Geometry: final body of the model. Coordinates: model frame, mm. Face numbers are marked on the shaded views. A direction names the side the tool comes from. Coordinates: 2 decimals unless noted, no trailing zeros. Write each loop counter-clockwise with the first axis right and the second up, starting at its lowest first coordinate (ties: lowest second). Pieces come first, ordered by that corner, then holes. Notation, with made-up numbers: (53.25, 65.25) - (72.25, 65.25) arc R9 cw to (72.25, 75.25) - close; hole circle Ø10 at (88.25, 8). An arc over 180 degrees is marked (long way). Answer as a JSON object with one key per item and string values. Group by question number.
Item 1: Section B-B on y = -16.25. Return loops of the section in (x, z), and give its area (3 significant figures).
Item 2: Section C-C on x = 32.5. Return loops of the section in (y, z).
Item 3: Line query: line 1 along Z through (x, y) = (21, -9); line 2 along Y through (x, z) = (87.5, 25); line 3 along X through (y, z) = (-10.25, 27.75). Output: solid intervals per line, ascending. Write a range as from..to.
Item 4: Section A-A on z = 7.5. Return loops of the section in (x, y).
Item 5: Set-up query: the marked faces 1, 2 and 3. Return all of +Z, -Z, +X, -X, +Y, -Y with unobstructed straight access to the full face (end or side cutting, diameter ignored); none if empty.
Item 6: First-contact query: pin 1 Ø4 at (x, y) = (32.5, -12.5) entering from +Z; pin 2 Ø2 at (x, z) = (44.5, 9) entering from -Y; pin 3 Ø3 at (x, z) = (65.5, 13) entering from -Y; pin 4 Ø10 at (y, z) = (-10, 22.5) entering from -X. Flat tips, straight axial feed; report the tip coordinate or a pass-through.
Item 7: Section D-D on z = 2.25. Return loops of the section in (x, y), and give its area (3 significant figures).
Item 8: Mould query, pull axis Z, two halves, no side actions, for the marked faces 4, 5 and 6. Classes: pulls with the +Z half, pulls with the -Z half, needs draft (parallel to the pull), parting line crosses it, or undercut.
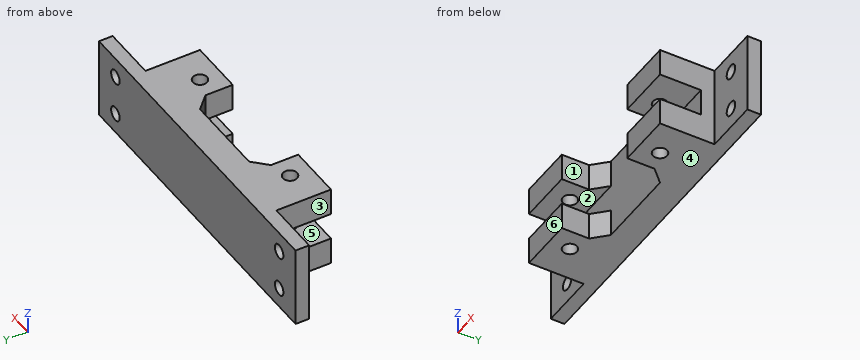
```python
from build123d import *

# Parameters (mm, degrees)
EXTRUDE_1_DEPTH     = 30
CHAMFER_2_SIZE      = 5
SKETCH_2_R          = 2.6
CUT_EXTRUDE_1_DEPTH = 127.194294641
SKETCH_3_W          = 10
SKETCH_3_H          = 15
CUT_EXTRUDE_2_DEPTH = 107.301458127
SKETCH_4_R          = 2.6
CUT_EXTRUDE_3_DEPTH = 126.299640861


with BuildPart() as part:
    # 草图1 → 凸台-拉伸1 (new body)
    with BuildSketch(Plane.XY):
        Polygon((20, 0), (20, -20), (40, -20), (40, -5), (80, -5), (80, -20), (100, -20), (100, 0), (120, 0), (120, 5), (0, 5), (0, 0), align=None)
    extrude(amount=EXTRUDE_1_DEPTH)

    # 倒角2
    chamfer_2_edges = [part.edges().sort_by_distance(p)[0] for p in [
        (80, -5, 15),
        (40, -5, 15),
    ]]
    chamfer(chamfer_2_edges, length=CHAMFER_2_SIZE)

    # 草图2 → 切除-拉伸1 (cut, through all)
    with BuildSketch(Plane(origin=(0, 5, 0), x_dir=(1, 0, 0), z_dir=(0, 1, 0))):
        with Locations(Location((10, -7.5, 0), (0, 0, 270))):
            Circle(SKETCH_2_R)
        with Locations(Location((10, -22.5, 0), (0, 0, 270))):
            Circle(SKETCH_2_R)
        with Locations(Location((110, -22.5, 0), (0, 0, 270))):
            Circle(SKETCH_2_R)
        with Locations(Location((110, -7.5, 0), (0, 0, 270))):
            Circle(SKETCH_2_R)
    extrude(amount=-CUT_EXTRUDE_1_DEPTH, mode=Mode.SUBTRACT)

    # 草图3 → 切除-拉伸2 (cut, through all)
    with BuildSketch(Plane.ZY.offset(-20)):
        with Locations((15, -12.5)):
            Rectangle(SKETCH_3_W, SKETCH_3_H)
    extrude(amount=-CUT_EXTRUDE_2_DEPTH, mode=Mode.SUBTRACT)

    # 草图4 → 切除-拉伸3 (cut, through all)
    with BuildSketch(Plane(origin=(0, 0, 0), x_dir=(-1, 0, 0), z_dir=(0, 0, -1))):
        with Locations((-87.5, -12.5)):
            Circle(SKETCH_4_R)
        with Locations((-32.5, -12.5)):
            Circle(SKETCH_4_R)
    extrude(amount=-CUT_EXTRUDE_3_DEPTH, mode=Mode.SUBTRACT)


solid = part.part
```
Checks:
{
 "1": {"outline": "(20, 0) - (40, 0) - (40, 10) - (20, 10) - close; (20, 20) - (40, 20) - (40, 30) - (20, 30) - close; (80, 0) - (100, 0) - (100, 10) - (80, 10) - close; (80, 20) - (100, 20) - (100, 30) - (80, 30) - close", "area": "800 mm^2"},
 "2": {"outline": "(-20, 0) - (-15.1, 0) - (-15.1, 10) - (-20, 10) - close; (-20, 20) - (-15.1, 20) - (-15.1, 30) - (-20, 30) - close; (-9.9, 0) - (5, 0) - (5, 30) - (-9.9, 30) - (-9.9, 20) - (-5, 20) - (-5, 10) - (-9.9, 10) - close"},
 "3": {"line 1": "0..10, 20..30", "line 2": "-20..-15.1, -9.9..5", "line 3": "20..31.2, 33.8..40, 80..86.2, 88.8..100"},
 "4": {"outline": "(0, 0) - (7.4, 0) - (7.4, 5) - (0, 5) - close; (12.6, 0) - (20, 0) - (20, -20) - (40, -20) - (40, -10) - (45, -5) - (75, -5) - (80, -10) - (80, -20) - (100, -20) - (100, 0) - (107.4, 0) - (107.4, 5) - (12.6, 5) - close; (112.6, 0) - (120, 0) - (120, 5) - (112.6, 5) - close; hole circle Ø5.2 at (32.5, -12.5); hole circle Ø5.2 at (87.5, -12.5)"},
 "5": {"face 1": "+Z, -Z, -Y", "face 2": "+X, -X, -Y", "face 3": "+Z, -Z, -X, -Y"},
 "6": {"pin 1": "through", "pin 2": "y = -6.5", "pin 3": "y = -5", "pin 4": "x = 20"},
 "7": {"outline": "(0, 0) - (20, 0) - (20, -20) - (40, -20) - (40, -10) - (45, -5) - (75, -5) - (80, -10) - (80, -20) - (100, -20) - (100, 0) - (120, 0) - (120, 5) - (0, 5) - close; hole circle Ø5.2 at (32.5, -12.5); hole circle Ø5.2 at (87.5, -12.5)", "area": "1,580 mm^2"},
 "8": {"face 4": "pulls with the -Z half", "face 5": "undercut", "face 6": "needs draft"}
}
